from build123d import *

# Parameters (mm, degrees)
F2_DEPTH  = 120
F3_W      = 36.2346663144
F3_H      = 240
F3_W_2    = 2.2
F3_H_2    = 235.6
F4_DEPTH  = 2
F5_R      = 2
F7_DEPTH  = 240
F8_W      = 15
F8_H      = 4.1411047216
F8_H_2    = 20.8588952784
F8_R      = 2
F9_DEPTH  = 3.3
F10_R     = 7.49999
F11_W     = 2.2
F11_H     = 25.02
F12_DEPTH = 2
F13_R     = 5
F14_R     = 7


# Not quite as in the source:
# - a fillet or chamfer is up to 0.001 mm smaller than in the source, because OpenCascade refuses the exact size
# - a feature names something its author has since deleted; it is built from what else it names


with BuildPart() as f2:
    # F1 (on Front) → F2 (new body, symmetric)
    with BuildSketch(Plane.XZ):
        Polygon((35, 11.4487740959), (0, 2.0705523608), (0, 0), (35, 9.3782217351), align=None)
    extrude(amount=F2_DEPTH, both=True)

    # F3 (on face) → F4 (join)
    with BuildSketch(Plane(origin=(0, 0, 0), x_dir=(0.9659258263, 0, 0.2588190451), z_dir=(0.2588190451, 0, -0.9659258263))):
        with Locations((18.1173331572, 0)):
            Rectangle(F3_W, F3_H)
        Polygon((2.2, -117.8), (2.2, 117.8), (6.4057777191, 117.8), (8.6057777191, 117.8), (17.0173331572, 117.8), (19.2173331572, 117.8), (27.6288885953, 117.8), (29.8288885953, 117.8), (34.0346663144, 117.8), (34.0346663144, -117.8), (29.8288885953, -117.8), (27.6288885953, -117.8), (19.2173331572, -117.8), (17.0173331572, -117.8), (8.6057777191, -117.8), (6.4057777191, -117.8), align=None, mode=Mode.SUBTRACT)
        with Locations((28.7288885953, 0)):
            Rectangle(F3_W_2, F3_H_2)
        with Locations((18.1173331572, 0)):
            Rectangle(F3_W_2, F3_H_2)
        with Locations((7.5057777191, 0)):
            Rectangle(F3_W_2, F3_H_2)
    extrude(amount=F4_DEPTH)

    # F5
    f5_edges = [f2.edges().sort_by_distance(p)[0] for p in [
        (33.133782, -117.8, 7.842894),
        (26.946276, -117.8, 6.184957),
        (16.696301, -117.8, 3.438484),
        (6.446325, -117.8, 0.692011),
        (29.071313, -117.8, 6.754359),
        (18.821337, -117.8, 4.007886),
        (8.571362, -117.8, 1.261413),
        (2.383856, -117.8, -0.396524),
        (2.383856, 117.8, -0.396524),
        (8.571362, 117.8, 1.261413),
        (18.821337, 117.8, 4.007886),
        (29.071313, 117.8, 6.754359),
        (33.133782, 117.8, 7.842894),
        (16.696301, 117.8, 3.438484),
        (6.446325, 117.8, 0.692011),
        (26.946276, 117.8, 6.184957),
    ]]
    fillet(f5_edges, radius=F5_R)

    # F6 (on face) → F7 (join, through all)
    with BuildSketch(Plane.XZ.offset(120)):
        Polygon((0, -2.0705523608), (0.5176380902, -1.9318516526), (0, 0), align=None)
    extrude(amount=-F7_DEPTH)

    # F8 (on face) → F9 (join)
    with BuildSketch(Plane(origin=(0, 0, 0), x_dir=(0, -1, 0), z_dir=(-1, 0, 0))):
        with Locations((-60, 0)):
            Rectangle(F8_W, F8_H)
        with Locations((-60, -12.5)):
            Rectangle(F8_W, F8_H_2)
        with Locations((-60, -15.9294476392)):
            Circle(F8_R, mode=Mode.SUBTRACT)
        with Locations((60, 0)):
            Rectangle(F8_W, F8_H)
        with Locations((60, -12.5)):
            Rectangle(F8_W, F8_H_2)
        with Locations((60, -15.9294476392)):
            Circle(F8_R, mode=Mode.SUBTRACT)
    extrude(amount=-F9_DEPTH)

    # F10 (radius 7.5 in the source; OpenCascade refuses exactly that, so slightly less here)
    f10_edges = [f2.edges().sort_by_distance(p)[0] for p in [
        (1.65, 67.5, -22.929448),
        (1.65, 52.5, -22.929448),
        (1.65, -52.5, -22.929448),
        (1.65, -67.5, -22.929448),
    ]]
    fillet(f10_edges, radius=F10_R)

    # F11 (on face) → F12 (join, through all)
    with BuildSketch(Plane(origin=(0.5176380902, 0, -1.9318516526), x_dir=(0.9659258263, 0, 0.2588190451), z_dir=(0.2588190451, 0, -0.9659258263))):
        Polygon((6.4057777191, -47.49), (2.2, -47.49), (2.2, -52.5), (2.2, -67.5), (2.2, -72.51), (6.4057777191, -72.51), align=None)
        with Locations((7.5057777191, -60)):
            Rectangle(F11_W, F11_H)
        Polygon((2.2, 52.5), (2.2, 47.49), (6.4057777191, 47.49), (6.4057777191, 72.51), (2.2, 72.51), (2.2, 67.5), align=None)
        with Locations((7.5057777191, 60)):
            Rectangle(F11_W, F11_H)
    extrude(amount=-F12_DEPTH)

    # F13
    f13_edges = [f2.edges().sort_by_distance(p)[0] for p in [
        (1.65, -52.5, -1.628436),
        (1.65, -67.5, -1.628436),
        (1.65, 52.5, -1.628436),
        (1.65, 67.5, -1.628436),
    ]]
    fillet(f13_edges, radius=F13_R)

    # F14
    f14_edges = [f2.edges().sort_by_distance(p)[0] for p in [
        (3.3, 60, -1.18632),
        (3.3, -60, -1.18632),
    ]]
    fillet(f14_edges, radius=F14_R)


solid = f2.part
CAD build for the part. Positions are in the model's coordinates, mm. A direction names the side the tool comes from. Coordinates: 2 decimals unless noted, no trailing zeros. Order: outer loops, then holes, each group sorted by start corner. A loop starts at its lowest first (then second) coordinate and runs counter-clockwise, first axis right, second up.
Item 1: Two-plate mould, pull along Z, no slides. Class faces 1 (the face through (1.673, -65.361, -20.674)), 2 (the face through (1.6, 58.1, -15.3)), 3 (the face through (3.3, 60, -13)): +Z half, -Z half, draft (parallel to the pull), parting line (faces both ways), or undercut.
Check sheet entries:
face 1: -Z half
face 2: undercut
face 3: draft
Item 2: Band-saw the part on A-A on y = 101.5. List the corners of the cut face in (x, z), plus the area to 3 significant figures.
Check sheet entries:
outline: (0, -2.07) - (2.64, -1.36) - (2.13, 0.57) - (6.19, 1.66) - (6.71, -0.27) - (8.83, 0.3) - (8.31, 2.23) - (16.44, 4.4) - (16.96, 2.47) - (19.08, 3.04) - (18.56, 4.97) - (26.69, 7.15) - (27.21, 5.22) - (29.33, 5.79) - (28.81, 7.72) - (32.87, 8.81) - (33.39, 6.88) - (35.52, 7.45) - (35, 9.38) - (35, 11.45) - (0, 2.07) - close
area: 95.0 mm2
Item 3: Pin check, flat tips, straight feed: pin 1 Ø6 at (y, z) = (-25, 7.5) entering from +X; pin 2 Ø1.7 at (x, z) = (1, -12) entering from +Y; pin 3 Ø12 at (y, z) = (59, -11.5) entering from +X; pin 4 Ø1.5 at (y, z) = (27.5, -4.5) entering from -X. Stop position of each tip, or through.
Check sheet entries:
pin 1: stops at x = 35.52
pin 2: stops at y = 67.5
pin 3: stops at x = 3.38
pin 4: passes through
Item 4: Drill centre lines: L1, parallel to Z at x = 2.2, y = -60; L2, parallel to X at y = -33, z = 0.5; L3, parallel to Z at x = 25, y = -6.5. Where is each one in solid material? Low to high.
Check sheet entries:
L1: z = -22.93 to -17.93, -13.93 to 2.66
L2: x = 0 to 2.14, 6.5 to 8.78
L3: z = 6.7 to 8.77
Item 5: 3-axis set-ups, long thin cutter, end or side, ignore diameter. For faces 4 (the face through (18, 120, 5)), 5 (the face through (3.3, -60, -13)), 6 (the face through (1.673, -54.755, -20.791)): which of +Z, -Z, +X, -X, +Y, -Y reach the whole face in a straight line?
Check sheet entries:
face 4: +Z, -Z, +X, -X, +Y
face 5: -Z, +X, +Y, -Y
face 6: -Z, +X, -X
